For this review, take the finished solid that the model builds, in its own axes (mm). Coordinates: 2 decimals unless noted, no trailing zeros. Write each loop counter-clockwise with the first axis right and the second up, starting at its lowest first coordinate (ties: lowest second). Pieces come first, ordered by that corner, then holes.
```python
from build123d import *

# Parameters (mm, degrees)
SKETCH1_W               = 812.8
SKETCH1_H               = 38.1
BOSS_EXTRUDE1_DEPTH     = 2.54
SKETCH2_R               = 12.7
CUT_EXTRUDE1_DEPTH      = 1
CUT_EXTRUDE1_DEPTH_BACK = 3.54


with BuildPart() as part:
    # Sketch1 → Boss-Extrude1 (new body)
    with BuildSketch(Plane(origin=(0, 0, 0), x_dir=(1, 0, 0), z_dir=(0, 1, 0))):
        Rectangle(SKETCH1_W, SKETCH1_H)
    extrude(amount=BOSS_EXTRUDE1_DEPTH)

    # Sketch2 → Cut-Extrude1 (cut, two sides)
    with BuildSketch(Plane(origin=(0, 2.54, 0), x_dir=(1, 0, 0), z_dir=(0, 1, 0))) as cut_extrude1_sk:
        with Locations((-384.175, 0)):
            Circle(SKETCH2_R)
        with Locations((384.175, 0)):
            Circle(SKETCH2_R)
    extrude(amount=CUT_EXTRUDE1_DEPTH, mode=Mode.SUBTRACT)
    extrude(cut_extrude1_sk.sketch, amount=-CUT_EXTRUDE1_DEPTH_BACK, mode=Mode.SUBTRACT)


solid = part.part
```
Q1. Draft analysis for pull direction Z (two halves, no side actions). For faces 1 (the cylindrical face through (396.29, 1.29, -3.81)), 2 (the flat face through (-6, 2.54, 0)), state which applies: +Z half, -Z half, draft (parallel to the pull), parting line (faces both ways), or undercut.
Ans:
face 1: undercut
face 2: draft
Q2. Add section B-B (y = 1.2). State the section outline as (x, z) points (3 decimals), then the cut area to 3 significant figures.
Ans:
outline: (-406.4, -19.05) - (406.4, -19.05) - (406.4, 19.05) - (-406.4, 19.05) - close; hole circle Ø25.4 at (-384.175, 0); hole circle Ø25.4 at (384.175, 0)
area: 30,000 mm2
Q3. For probe 1 along X at (y, z) = (1.9, 0) (3 decimals); probe 2 along X at (y, z) = (1.8, -2.5), list the stretches that pass through material, from the lowest coordinate up.
Ans:
probe 1: x = -406.4 to -396.875, -371.475 to 371.475, 396.875 to 406.4
probe 2: x = -406.4 to -396.63, -371.72 to 371.72, 396.63 to 406.4
Q4. Add section A-A (z = 0). State the section outline as (x, y) points (3 decimals).
Ans:
outline: (-406.4, 0) - (-396.875, 0) - (-396.875, 2.54) - (-406.4, 2.54) - close; (-371.475, 0) - (371.475, 0) - (371.475, 2.54) - (-371.475, 2.54) - close; (396.875, 0) - (406.4, 0) - (406.4, 2.54) - (396.875, 2.54) - close
